Model file for the job. Use its own axes, mm. Face numbers are marked on the shaded views. A direction names the side the tool comes from. Coordinates: 2 decimals unless noted, no trailing zeros. Order: outer loops, then holes, each group sorted by start corner. A loop starts at its lowest first (then second) coordinate and runs counter-clockwise, first axis right, second up.
from build123d import *

# Parameters (mm, degrees)
F0_R     = 1.5875
F0_R_2   = 4.7625
F1_DEPTH = 6.35
F2_R     = 2.54


# Not quite as in the source:
# - a length typed as a fraction of an inch, garbled in the dataset ("3 / 203.2 mm" for 3/8 in), is restored


with BuildPart() as f1:
    # F0 (on Top) → F1 (new body)
    with BuildSketch(Plane.XY):
        with BuildLine():
            Line((3.175, -22.440738686), (0, -27.94))
            Line((0, -27.94), (-3.175, -22.440738686))
            Line((-3.175, -22.440738686), (-3.175, -47.840738686))
            ThreePointArc((-3.175, -47.840738686), (0, -51.015738686), (3.175, -47.840738686))
            Line((3.175, -47.840738686), (3.175, -22.440738686))
        make_face()
        with Locations((0, -47.840738686)):
            Circle(F0_R, mode=Mode.SUBTRACT)
        Polygon((-3.175, -22.440738686), (0, -27.94), (3.175, -22.440738686), (21.0217497817, 8.470738686), (24.1967497817, 13.97), (17.8467497817, 13.97), (-17.8467497817, 13.97), (-24.1967497817, 13.97), (-21.0217497817, 8.470738686), align=None)
        with Locations((0, -21.59)):
            Circle(F0_R, mode=Mode.SUBTRACT)
        with Locations((0, -12.7)):
            Circle(F0_R_2, mode=Mode.SUBTRACT)
        Circle(F0_R_2, mode=Mode.SUBTRACT)
        with Locations((-10.9985226281, 6.35)):
            Circle(F0_R_2, mode=Mode.SUBTRACT)
        with Locations((-18.6974884677, 10.795)):
            Circle(F0_R, mode=Mode.SUBTRACT)
        with Locations((10.9985226281, 6.35)):
            Circle(F0_R_2, mode=Mode.SUBTRACT)
        with Locations((18.6974884677, 10.795)):
            Circle(F0_R, mode=Mode.SUBTRACT)
        with BuildLine():
            Line((-43.0187950379, 21.170738686), (-21.0217497817, 8.470738686))
            Line((-21.0217497817, 8.470738686), (-24.1967497817, 13.97))
            Line((-24.1967497817, 13.97), (-17.8467497817, 13.97))
            Line((-17.8467497817, 13.97), (-39.8437950379, 26.67))
            ThreePointArc((-39.8437950379, 26.67), (-44.1809256949, 25.507869343), (-43.0187950379, 21.170738686))
        make_face()
        with Locations((-41.4312950379, 23.920369343)):
            Circle(F0_R, mode=Mode.SUBTRACT)
        with BuildLine():
            Line((24.1967497817, 13.97), (21.0217497817, 8.470738686))
            Line((21.0217497817, 8.470738686), (43.0187950379, 21.170738686))
            ThreePointArc((43.0187950379, 21.170738686), (44.1809256949, 25.507869343), (39.8437950379, 26.67))
            Line((39.8437950379, 26.67), (17.8467497817, 13.97))
            Line((17.8467497817, 13.97), (24.1967497817, 13.97))
        make_face()
        with Locations((41.4312950379, 23.920369343)):
            Circle(F0_R, mode=Mode.SUBTRACT)
    extrude(amount=F1_DEPTH)

    # F2
    f2_edges = [f1.edges().sort_by_distance(p)[0] for p in [
        (-3.175, -22.440739, 3.175),
        (-21.02175, 8.470739, 3.175),
        (-17.84675, 13.97, 3.175),
        (17.84675, 13.97, 3.175),
        (21.02175, 8.470739, 3.175),
        (3.175, -22.440739, 3.175),
    ]]
    fillet(f2_edges, radius=F2_R)


solid = f1.part
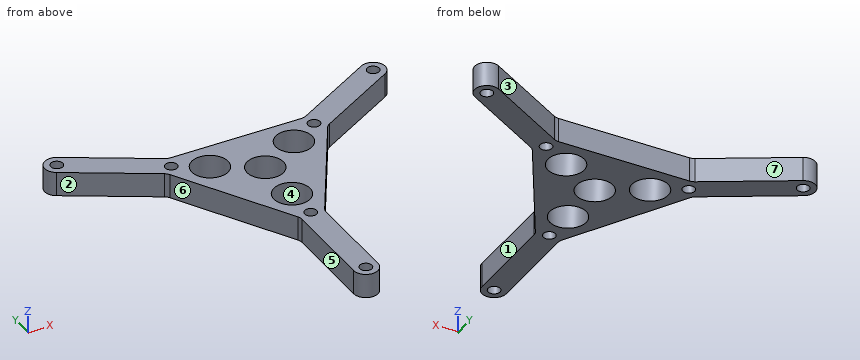
Q1. Drop flat-ended pins along their axis: P1, Ø2.5, axis at x = -18.7, y = 10.8, coming from the +Z side; P2, Ø11, axis at x = -11, y = 6.35, coming from the +Z side. Give the stop position or say it passes through.
Established:
P1: passes through
P2: stops at z = 6.35
Q2. Mould opens along Y. For the marked faces 4, 5, 6 and 7 say: pulls with the +Y half, pulls with the -Y half, needs draft (parallel to the pull), parting line crosses it, or undercut.
Established:
face 4: undercut
face 5: needs draft
face 6: pulls with the -Y half
face 7: pulls with the +Y half
Q3. Cut at A-A, the plane x = 0. List the corners of the cut face in (y, z), plus the area to 3 significant figures.
Established:
outline: (-51.02, 0) - (-49.43, 0) - (-49.43, 6.35) - (-51.02, 6.35) - close; (-46.25, 0) - (-23.18, 0) - (-23.18, 6.35) - (-46.25, 6.35) - close; (-20, 0) - (-17.46, 0) - (-17.46, 6.35) - (-20, 6.35) - close; (-7.94, 0) - (-4.76, 0) - (-4.76, 6.35) - (-7.94, 6.35) - close; (4.76, 0) - (13.97, 0) - (13.97, 6.35) - (4.76, 6.35) - close
area: 251 mm2
Q4. Cut at B-B, the plane y = -12.7. List the corners of the cut face in (x, z), plus the area to 3 significant figures.
Established:
outline: (-8.8, 0) - (-4.76, 0) - (-4.76, 6.35) - (-8.8, 6.35) - close; (4.76, 0) - (8.8, 0) - (8.8, 6.35) - (4.76, 6.35) - close
area: 51.3 mm2
Q5. Probe line 1 (Y direction, x = 0, z = 2); line 2 (Y direction, x = 2, z = 3.75); line 3 (X direction, y = -23.5, z = 3) (3 decimals). List the from-to ranges inside material, lowest first.
Established:
line 1: y = -51.02 to -49.43, -46.25 to -23.18, -20 to -17.46, -7.94 to -4.76, 4.76 to 13.97
line 2: y = -50.31 to -17.02, -8.38 to -4.32, 4.32 to 13.97
line 3: x = -3.175 to 3.175
Q6. Which spindle directions (+Z, -Z, +X, -X, +Y, -Y) get a long thin tool onto all of the face, cutting with end or side? Do the marked faces 1, 2 and 3. Say none if no direction does.
Established:
face 1: +Z, -Z, +X, -Y
face 2: +Z, -Z, -X, -Y
face 3: +Z, -Z, +Y
Q7. Cut at C-C, the plane z = 1.75. Count the separate pieces of the cut face and the enclosed holes in it, plus the area to 3 significant figures.
Established:
separate pieces: 1
enclosed holes: 10
area: 1,160 mm2
Q8. Cut at D-D, the plane y = 19.5. List the corners of the cut face in (x, z) (3 decimals), plus the area to 3 significant figures.
Established:
outline: (-40.125, 0) - (-27.425, 0) - (-27.425, 6.35) - (-40.125, 6.35) - close; (27.425, 0) - (40.125, 0) - (40.125, 6.35) - (27.425, 6.35) - close
area: 161 mm2
